Source: CAD feature listing. Evaluate the final solid. Frame: model axes, mm. Face numbers are marked on the shaded views. A direction names the side the tool comes from. Give positions to 0.01 mm unless a question says otherwise; leave off trailing zeros. Order: outer loops, then holes, each group sorted by start corner. A loop starts at its lowest first (then second) coordinate and runs counter-clockwise, first axis right, second up.
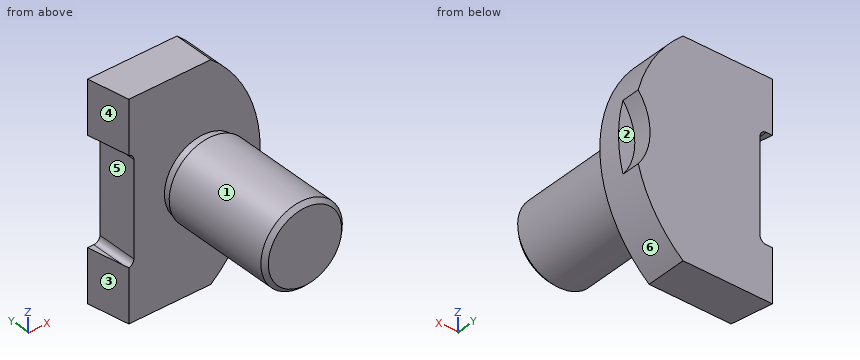
from build123d import *

# Parameters (mm, degrees)
SKETCH_1_R               = 10
EXTRUDE_1_DEPTH          = 40
CHAMFER_1_SIZE           = 1
EXTRUDE_2_DEPTH          = 10
SKETCH_3_R               = 14
CUT_EXTRUDE_1_DEPTH      = 4.5
CUT_EXTRUDE_2_DEPTH      = 69.585712798
CUT_EXTRUDE_2_DEPTH_BACK = 69.585712798
SKETCH_5_OUTSIDE_W       = 50.778
SKETCH_5_OUTSIDE_H       = 68.778
SKETCH_5_OUTSIDE_R       = 9.5
CUT_EXTRUDE_3_DEPTH      = 2
FILLET_1_R               = 1.5


with BuildPart() as part:
    # 草图1 → 凸台-拉伸1 (new body)
    with BuildSketch(Plane(origin=(0, 0, 0), x_dir=(1, 0, 0), z_dir=(0, 1, 0))):
        with Locations(Location((0, 0, 0), (0, 0, 270))):
            Circle(SKETCH_1_R)
    extrude(amount=EXTRUDE_1_DEPTH)

    # 倒角1
    chamfer_1_edges = [part.edges().sort_by_distance(p)[0] for p in [
        (0, 0, -10),
    ]]
    chamfer(chamfer_1_edges, length=CHAMFER_1_SIZE)

    # 草图2 → 凸台-拉伸2 (add)
    with BuildSketch(Plane(origin=(0, 40, 0), x_dir=(1, 0, 0), z_dir=(0, 1, 0))):
        with BuildLine():
            Line((-17, -13), (-17, 13))
            Line((-17, 13), (-20, 13))
            Line((-20, 13), (-20, 26))
            Line((-20, 26), (1.9089023, 26))
            ThreePointArc((1.9089023, 26), (14, 0), (1.9089023, -26))
            Line((1.9089023, -26), (-20, -26))
            Line((-20, -26), (-20, -13))
            Line((-20, -13), (-17, -13))
        make_face()
    extrude(amount=-EXTRUDE_2_DEPTH)

    # 草图3 → 切除-拉伸1 (cut)
    with BuildSketch(Plane(origin=(0, 40, 0), x_dir=(1, 0, 0), z_dir=(0, 1, 0))):
        with Locations((24, 0)):
            Circle(SKETCH_3_R)
    extrude(amount=-CUT_EXTRUDE_1_DEPTH, mode=Mode.SUBTRACT)

    # 草图4 → 切除-拉伸2 (cut, two sides: drawn at the far end of the back side and taken through both)
    with BuildSketch(Plane.XY.offset(26).offset(-CUT_EXTRUDE_2_DEPTH_BACK)):
        Polygon((-39.968713517, 153.248201929), (-20, 40), (-18.236730193, 30), (1.731983324, -83.248201929), (-224.764420535, -123.185628963), (-266.465117376, 113.310774896), align=None)
    extrude(amount=CUT_EXTRUDE_2_DEPTH + CUT_EXTRUDE_2_DEPTH_BACK, mode=Mode.SUBTRACT)

    # 草图5 outside → 切除-拉伸3 (cut)
    with BuildSketch(Plane.XZ.offset(-30)):
        with Locations((-3, 0)):
            Rectangle(SKETCH_5_OUTSIDE_W, SKETCH_5_OUTSIDE_H)
        with Locations(Location((0, 0, 0), (0, 0, 270))):
            Circle(SKETCH_5_OUTSIDE_R, mode=Mode.SUBTRACT)
    extrude(amount=CUT_EXTRUDE_3_DEPTH, mode=Mode.SUBTRACT)

    # 圆角1
    fillet_1_edges = [part.edges().sort_by_distance(p)[0] for p in [
        (-17, 35, 13),
        (-17, 35, -13),
    ]]
    fillet(fillet_1_edges, radius=FILLET_1_R)


solid = part.part
1) Section query C-C on x = 11. Output: boundary loops of the cut face in (y, z), and give its area (3 significant figures).
Checks:
outline: (30, -13.96) - (40, -13.96) - (40, -5.2) - (35.5, -5.2) - (35.5, 5.2) - (40, 5.2) - (40, 13.96) - (30, 13.96) - close
area: 233 mm2
2) Pull-direction query (Z, two-part tool) for the marked faces 4, 5 and 6; classes: +Z half, -Z half, draft (parallel to the pull), parting line (faces both ways), or undercut.
Checks:
face 4: draft
face 5: undercut
face 6: parting line
3) Section query A-A on z = 0. Output: boundary loops of the cut face in (x, y), and give its area (3 significant figures).
Checks:
outline: (-17, 30) - (-9.5, 30) - (-9.5, 28) - (-10, 28) - (-10, 1) - (-9, 0) - (9, 0) - (10, 1) - (10, 28) - (9.5, 28) - (9.5, 30) - (14, 30) - (14, 35.5) - (10, 35.5) - (10, 40) - (-17, 40) - close
area: 889 mm2
4) Reachability of the marked faces 1, 2 and 3 from +Z, -Z, +X, -X, +Y, -Y: full face, straight path, thin tool, end or side. Return the list, or none.
Checks:
face 1: -Y
face 2: +X, +Y
face 3: +Z, -Z, -X, -Y
5) Ray query, L1, parallel to Y at x = -5, z = -19.5; L2, parallel to X at y = 22, z = 0; L3, parallel to Y at x = 1.5, z = -9.5. Return the intervals inside material, ascending.
Checks:
L1: y = 30 to 40
L2: x = -10 to 10
L3: y = 0.62 to 28, 30 to 40
6) Section query D-D on z = -18.5. Output: boundary loops of the cut face in (x, y).
Checks:
outline: (-20, 40) - (-18.24, 30) - (8.53, 30) - (8.53, 40) - close
7) First-contact query: pin 1 Ø8 at (x, z) = (-4, 17) entering from -Y; pin 2 Ø12 at (x, y) = (6, 18) entering from -Z; pin 3 Ø6 at (x, y) = (10, 21) entering from -Z. Flat tips, straight axial feed; report the tip coordinate or a pass-through.
Checks:
pin 1: stops at y = 30
pin 2: stops at z = -10
pin 3: stops at z = -7.14
8) Section query B-B on x = 0. Output: boundary loops of the cut face in (y, z), and give its area (3 significant figures).
Checks:
outline: (0, -9) - (1, -10) - (28, -10) - (28, -9.5) - (30, -9.5) - (30, -26) - (40, -26) - (40, 26) - (30, 26) - (30, 9.5) - (28, 9.5) - (28, 10) - (1, 10) - (0, 9) - close
area: 1,120 mm2
